```python
from build123d import *

# Parameters (mm, degrees)
F1_DEPTH = 3
F2_DEPTH = 2.5
F3_R     = 1.75
F4_DEPTH = 3.001
F5_R     = 3.5
F6_DEPTH = 1
F7_R     = 5.08


with BuildPart() as f1:
    # F0 (on Top) → F1 (new body)
    with BuildSketch(Plane.XY):
        Polygon((15, 15), (25, 25), (-25, 25), (-25, -25), (-15, -15), (-15, 15), align=None)
    extrude(amount=F1_DEPTH)

    # F0 (on Top) → F2 (join)
    with BuildSketch(Plane.XY):
        Polygon((-15, -15), (15, 15), (-15, 15), align=None)
    extrude(amount=F2_DEPTH)

    # F3 (on face) → F4 (cut, through all)
    with BuildSketch(Plane.XY.offset(3)):
        with Locations((-20, 20)):
            Circle(F3_R)
        with Locations((0, 20)):
            Circle(F3_R)
        with Locations((-20, 0)):
            Circle(F3_R)
    extrude(amount=-F4_DEPTH, mode=Mode.SUBTRACT)

    # F5 (on face) → F6 (cut)
    with BuildSketch(Plane.XY):
        with Locations((-20, 0)):
            Circle(F5_R)
        with Locations((-20, 20)):
            Circle(F5_R)
        with Locations((0, 20)):
            Circle(F5_R)
    extrude(amount=F6_DEPTH, mode=Mode.SUBTRACT)

    # F7
    f7_edges = [f1.edges().sort_by_distance(p)[0] for p in [
        (25, 25, 1.5),
        (-25, -25, 1.5),
        (-25, 25, 1.5),
    ]]
    fillet(f7_edges, radius=F7_R)


solid = f1.part
```
Model file for the job. Use its own axes, mm. A direction names the side the tool comes from. Give positions to 0.01 mm unless a question says otherwise; leave off trailing zeros. Loops run counter-clockwise (first coordinate to the right, second up) from the corner with the lowest first, then second, coordinate; pieces in that order, holes last. Notation, with made-up numbers: (-30, -35.75) - (-9, -35.75) arc R24 cw to (-9, -13.75) - close; hole circle Ø8 at (52.5, -4). An arc over 180 degrees is marked (long way). One line per item, written item: value. Start each with the question number.
1. Slice it at D-D (x = -17.5). List the corners of the cut face in (y, z), plus the area to 3 significant figures.
2. Slice it at C-C (y = -7). List the corners of the cut face in (x, z).
3. Pin check, flat tips, straight feed: pin 1 (2 mm diameter, centred on x = -19.5, y = 1.5, fed in from -Z); pin 2 (3 mm diameter, centred on x = -20, y = 20, fed in from +Z); pin 3 (9 mm diameter, centred on x = -1, y = -2, fed in from +Z); pin 4 (1 mm diameter, centred on y = -4, z = 2, fed in from +X). Stop position of each tip, or through.
4. Which spindle directions (+Z, -Z, +X, -X, +Y, -Y) get a long thin tool onto all of the face, cutting with end or side? Do faces 4 (the flat face through (-4, 4, 2.5)), 5 (the cylindrical face through (-18.12, 22.95, 0.49)), 6 (the flat face through (-3, 25, 1)). Say none if no direction does.
5. Slice it at B-B (y = 0). List the corners of the cut face in (x, z), plus the area to 3 significant figures.
6. Slice it at A-A (x = 0). List the corners of the cut face in (y, z), plus the area to 3 significant figures.
7. Probe L1, parallel to Y at x = -20, z = 0.7; L2, parallel to Y at x = -20, z = 2; L3, parallel to Z at x = -0.5, y = 22. List the from-to ranges inside material, lowest first. Write a range as from..to.
8. Pull direction Y, two halves, no side cores. Call faces 1 (the cylindrical face through (-23.551, 23.472, 1.521)), 2 (the flat face through (-22, -1, 1)), 3 (the flat face through (-13, 18, 3)): pulls with the +Y half, pulls with the -Y half, needs draft (parallel to the pull), parting line crosses it, or undercut.
Solution:
1. outline: (-17.2, 0) - (-2.45, 0) - (-2.45, 1) - (2.45, 1) - (2.45, 0) - (17.55, 0) - (17.55, 1) - (22.45, 1) - (22.45, 0) - (25, 0) - (25, 3) - (-17.2, 3) - close
1. area: 117 mm^2
2. outline: (-25, 0) - (-7, 0) - (-7, 2.5) - (-15, 2.5) - (-15, 3) - (-25, 3) - close
3. pin 1: stops at z = 1
3. pin 2: passes through
3. pin 3: stops at z = 2.5
3. pin 4: stops at x = -3.5
4. face 4: +Z, +X, -Y
4. face 5: -Z
4. face 6: +Z, -Z, +X, -X, +Y
5. outline: (-25, 0) - (-23.5, 0) - (-23.5, 1) - (-21.75, 1) - (-21.75, 3) - (-25, 3) - close; (-18.25, 1) - (-16.5, 1) - (-16.5, 0) - (0, 0) - (0, 2.5) - (-15, 2.5) - (-15, 3) - (-18.25, 3) - close
5. area: 53.5 mm^2
6. outline: (0, 0) - (16.5, 0) - (16.5, 1) - (18.25, 1) - (18.25, 3) - (15, 3) - (15, 2.5) - (0, 2.5) - close; (21.75, 1) - (23.5, 1) - (23.5, 0) - (25, 0) - (25, 3) - (21.75, 3) - close
6. area: 53.5 mm^2
7. L1: y = -17.82..-3.5, 3.5..16.5, 23.5..25
7. L2: y = -17.82..-1.75, 1.75..18.25, 21.75..25
7. L3: z = 1..3
8. face 1: pulls with the +Y half
8. face 2: undercut
8. face 3: needs draft
